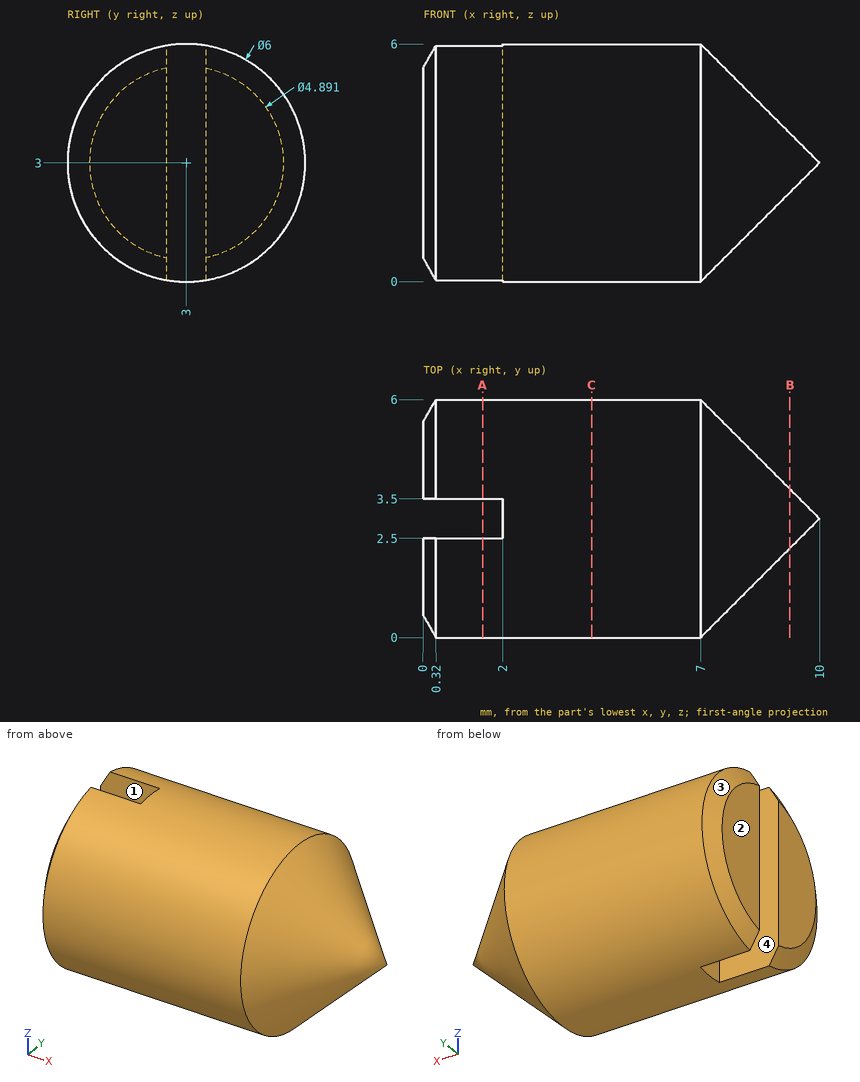
Part print with two shaded views. Sizes in mm from the minimum x, y, z corner. Round coordinates to 2 decimals unless told otherwise and drop trailing zeros. Write each loop counter-clockwise with the first axis right and the second up, starting at its lowest first coordinate (ties: lowest second). Pieces come first, ordered by that corner, then holes. Notation, with made-up numbers: M -6,71.25 L 12,71.25 A15 ccw 12,90.25 Z; hole C 40,52 d8. An arc over 180 degrees is marked long. Use CSV: the item, a comma, the result in double quotes.
1. Flat gauge pins, fed straight in: pin 1 (0.6 mm diameter, centred on x = 1, z = 3.5, fed in from -Y); pin 2 (2 mm diameter, centred on y = 2.5, z = 1, fed in from +X). Where does each tip first touch, or does it go through?
Reply:
pin 1,"stops at y = 0.01"
pin 2,"stops at x = 8.94"
2. Saw through at A-A (x = 1.5). Give the cut face in (y, z).
Reply:
outline,"M 2.5,0.04 L 2.5,5.96 A3 ccw Z; M 3.5,0.04 A3 ccw 3.5,5.96 Z"
3. Wall check: probe 1 along Y at (x, z) = (0.75, 2.25) (1 decimal); probe 2 along Y at (x, z) = (1, 2.75); probe 3 along X at (y, z) = (2.15, 3.5). Give the ranges that are in metal, low to high. Write a range as from..to.
Reply:
probe 1,"y = 0.1..2.5, 3.5..5.9"
probe 2,"y = 0.01..2.5, 3.5..5.99"
probe 3,"x = 0..9.01"
4. Two-plate mould, pull along Y, no slides. Class the marked faces 1, 2, 3 and 4: +Y half, -Y half, draft (parallel to the pull), parting line (faces both ways), or undercut.
Reply:
face 1,"undercut"
face 2,"draft"
face 3,"+Y half"
face 4,"undercut"
5. Saw through at C-C (x = 4.25). Give the cut face in (y, z).
Reply:
outline,"C 3,3 d6"
6. Saw through at B-B (x = 9.25). Give the cut face in (y, z).
Reply:
outline,"C 3,3 d1.5"
